```python
from build123d import *

# Parameters (mm, degrees)
SKETCH_1_R          = 35
SKETCH_1_R_2        = 3
EXTRUDE_1_DEPTH     = 6
SKETCH_3_R          = 3
CUT_EXTRUDE_2_DEPTH = 50.859803449
SKETCH_4_R          = 2
EXTRUDE_2_DEPTH     = 22
SKETCH_7_R          = 4
EXTRUDE_3_DEPTH     = 2
CHAMFER_1_SIZE      = 1
CUT_EXTRUDE_START   = -0.5
SKETCH_9_W          = 2
SKETCH_9_H          = 2
CUT_EXTRUDE_5_DEPTH = 4
FILLET_1_R          = 0.1
SKETCH_12_R         = 4
CUT_EXTRUDE_6_DEPTH = 2
CUT_EXTRUDE_START_2 = -2.5
SKETCH_13_R         = 2
SKETCH_13_R_2       = 1.9
CUT_EXTRUDE_7_DEPTH = 0.5


with BuildPart() as part:
    # 草图1 → 凸台-拉伸1 (new body)
    with BuildSketch(Plane.XY):
        Circle(SKETCH_1_R)
        Circle(SKETCH_1_R_2, mode=Mode.SUBTRACT)
    extrude(amount=EXTRUDE_1_DEPTH)

    # 草图3 → 切除-拉伸2 (cut, through all)
    with BuildSketch(Plane(origin=(0, 0, 0), x_dir=(-1, 0, 0), z_dir=(0, 0, -1))):
        with Locations((-4.582105158, 17.407019053)):
            Circle(SKETCH_3_R)
        with Locations((9.068583583, 15.548658842)):
            Circle(SKETCH_3_R)
        with Locations((17.407019053, 4.582105158)):
            Circle(SKETCH_3_R)
        with Locations((15.548658842, -9.068583583)):
            Circle(SKETCH_3_R)
        with Locations((4.582105158, -17.407019053)):
            Circle(SKETCH_3_R)
        with Locations((-9.068583583, -15.548658842)):
            Circle(SKETCH_3_R)
        with Locations((-17.407019053, -4.582105158)):
            Circle(SKETCH_3_R)
        with Locations((-15.548658842, 9.068583583)):
            Circle(SKETCH_3_R)
    extrude(amount=-CUT_EXTRUDE_2_DEPTH, mode=Mode.SUBTRACT)

    # 草图4 → 凸台-拉伸2 (add)
    with BuildSketch(Plane.XY.offset(6)):
        with Locations((9.178670771, -3.968879298)):
            Circle(SKETCH_4_R)
    extrude(amount=EXTRUDE_2_DEPTH)

    # 草图7 → 凸台-拉伸3 (add)
    with BuildSketch(Plane.XY.offset(28)):
        with Locations((9.178670771, -3.968879298)):
            Circle(SKETCH_7_R)
    extrude(amount=-EXTRUDE_3_DEPTH)

    # 倒角1
    chamfer_1_edges = [part.edges().sort_by_distance(p)[0] for p in [
        (7.178670771, -3.968879298, 6),
    ]]
    chamfer(chamfer_1_edges, length=CHAMFER_1_SIZE)

    # 草图9 → 切除-拉伸5 (cut)
    with BuildSketch(Plane.XY.offset(6).offset(CUT_EXTRUDE_START)):
        with Locations((0, -3)):
            Rectangle(SKETCH_9_W, SKETCH_9_H)
    extrude(amount=-CUT_EXTRUDE_5_DEPTH, mode=Mode.SUBTRACT)

    # 圆角1
    fillet_1_edges = [part.edges().sort_by_distance(p)[0] for p in [
        (1, -4, 3.5),
        (-1, -4, 3.5),
    ]]
    fillet(fillet_1_edges, radius=FILLET_1_R)

    # 草图12 → 切除-拉伸6 (cut)
    with BuildSketch(Plane.XY.offset(28)):
        with Locations((9.178670771, -3.968879298)):
            Circle(SKETCH_12_R)
    extrude(amount=-CUT_EXTRUDE_6_DEPTH, mode=Mode.SUBTRACT)

    # 草图13 → 切除-拉伸7 (cut)
    with BuildSketch(Plane.XY.offset(26).offset(CUT_EXTRUDE_START_2)):
        with Locations((9.178670771, -3.968879298)):
            Circle(SKETCH_13_R)
        with Locations((9.178670771, -3.968879298)):
            Circle(SKETCH_13_R_2, mode=Mode.SUBTRACT)
    extrude(amount=CUT_EXTRUDE_7_DEPTH, mode=Mode.SUBTRACT)


solid = part.part
```
CAD build for the part. Positions are in the model's coordinates, mm. A direction names the side the tool comes from. Round coordinates to 2 decimals unless told otherwise and drop trailing zeros. Write each loop counter-clockwise with the first axis right and the second up, starting at its lowest first coordinate (ties: lowest second). Pieces come first, ordered by that corner, then holes. Notation, with made-up numbers: (87.25, 0.5) -> (103.25, 0.5) arc R13 cw to (103.25, 21.5) -> close; hole circle Ø8 at (46, -23). An arc over 180 degrees is marked (long way). Answer in a Markdown table with one row per item. Add a question column.
Item 1: Drop flat-ended pins along their axis: pin 1 Ø3 at (x, y) = (24, -1) entering from +Z; pin 2 Ø8 at (x, z) = (7, 20.5) entering from -Y; pin 3 Ø5 at (x, y) = (15.55, 9.07) entering from +Z; pin 4 Ø1.2 at (y, z) = (-3, 3) entering from -X. Give the stop position or say it passes through.
Item 2: Drill centre lines: line 1 (X direction, y = -7, z = 3); line 2 (Y direction, x = 0, z = 2.35); line 3 (X direction, y = -4, z = 17.5). Where is each one in solid material? Low to high. Write a range as from..to.
Item 3: Saw through at C-C, the plane x = -16. Write the cut outline in (y, z).
Item 4: Saw through at A-A, the plane y = 0. Write the cut outline in (x, z).
Item 5: Which spindle directions (+Z, -Z, +X, -X, +Y, -Y) get a long thin tool onto all of the face, cutting with end or side? Do faces 4 (the face through (7.18, -3.88, 15.13)), 5 (the face through (18.1, -7.5, 3)). Say none if no direction does.
Item 6: Mould opens along Z. For faces 1 (the face through (0, -7, 6)), 2 (the face through (-28, -21, 3)), 3 (the face through (0, -4, 4)) say: pulls with the +Z half, pulls with the -Z half, needs draft (parallel to the pull), parting line crosses it, or undercut.
Item 7: Saw through at B-B, the plane x = 0. Write the cut outline in (y, z), then the cut area to 3 significant figures.
Item 8: Saw through at D-D, the plane z = 4.25. Count the separate pieces of the cut face and the enclosed holes in it, then the cut area to 3 significant figures.
Findings below:
| question | item | result |
|---|---|---|
| 1 | pin 1 | stops at z = 6 |
| 1 | pin 2 | stops at y = -5.97 |
| 1 | pin 3 | passes through |
| 1 | pin 4 | stops at x = -34.92 |
| 2 | line 1 | x = -34.29..-17.72, -13.38..15.63, 19.18..34.29 |
| 2 | line 2 | y = -35..-4, 3..35 |
| 2 | line 3 | x = 7.18..11.18 |
| 3 | outline | (-31.13, 0) -> (-12.03, 0) -> (-12.03, 6) -> (-31.13, 6) -> close; (-6.1, 0) -> (1.93, 0) -> (1.93, 6) -> (-6.1, 6) -> close; (7.23, 0) -> (31.13, 0) -> (31.13, 6) -> (7.23, 6) -> close |
| 4 | outline | (-35, 0) -> (-3, 0) -> (-3, 6) -> (-35, 6) -> close; (3, 0) -> (35, 0) -> (35, 6) -> (3, 6) -> close |
| 5 | face 4 | +Z |
| 5 | face 5 | +Z, -Z |
| 6 | face 1 | pulls with the +Z half |
| 6 | face 2 | needs draft |
| 6 | face 3 | undercut |
| 7 | outline | (-35, 0) -> (-3, 0) -> (-3, 1.5) -> (-4, 1.5) -> (-4, 5.5) -> (-3, 5.5) -> (-3, 6) -> (-35, 6) -> close; (3, 0) -> (35, 0) -> (35, 6) -> (3, 6) -> close |
| 7 | area | 380 mm^2 |
| 8 | separate pieces | 1 |
| 8 | enclosed holes | 9 |
| 8 | area | 3,590 mm^2 |
